```python
from build123d import *

# Parameters (mm, degrees)
F1_ANGLE      = 30
F2_R          = 3.81
F3_DEPTH      = 151.131
F3_DEPTH_BACK = 151.131
F4_W          = 5.08
F4_H          = 20.3206839475
F5_DEPTH      = 2.54


with BuildPart() as f1:
    # F0 (on Top) → F1 (revolve)
    with BuildSketch(Plane.XY):
        with BuildLine():
            Line((-151.13, 0), (-146.05, 0))
            ThreePointArc((-146.05, 0), (0, 146.05), (146.05, 0))
            Line((146.05, 0), (151.13, 0))
            ThreePointArc((151.13, 0), (0, 151.13), (-151.13, 0))
        make_face()
    revolve(axis=Axis((-73.025, 0, 0), (1, 0, 0)), revolution_arc=F1_ANGLE)

    # F2 (on Right) → F3 (cut, two sides)
    with BuildSketch(Plane.YZ) as f3_sk:
        Circle(F2_R)
    extrude(amount=-F3_DEPTH, mode=Mode.SUBTRACT)
    extrude(f3_sk.sketch, amount=F3_DEPTH_BACK, mode=Mode.SUBTRACT)

    # F4 (on Top) → F5 (join)
    with BuildSketch(Plane.XY):
        with Locations((0, 148.5682533469)):
            Rectangle(F4_W, F4_H)
    extrude(amount=F5_DEPTH)


solid = f1.part
```
Work out the finished part from the listing and answer in its coordinate system (mm). Coordinates: 2 decimals unless noted, no trailing zeros. Loops run counter-clockwise (first coordinate to the right, second up) from the corner with the lowest first, then second, coordinate; pieces in that order, holes last. Notation, with made-up numbers: (41.25, 70) - (81.25, 70) arc R33 ccw to (81.25, 107) - close; hole circle Ø2 at (15, -37.75). An arc over 180 degrees is marked (long way). Use a Markdown table: item, result.
Item 1: The mould has two halves that part along Z. Classify faces 1 (the flat face through (-34.279, 124.092, 71.645)), 2 (the flat face through (-1, 139, 0)): +Z half, -Z half, draft (parallel to the pull), parting line (faces both ways), or undercut.
Evaluation:
| item | result |
|---|---|
| face 1 | +Z half |
| face 2 | -Z half |
Item 2: Find section B-B, the plane y = 78. Determine the outline of the cut face in (x, z), and give its area (3 significant figures).
Evaluation:
| item | result |
|---|---|
| outline | (-129.45, 0) - (-123.48, 0) arc R123.48 cw to (-114.97, 45.03) - (-121.36, 45.03) arc R129.45 ccw to start; (114.97, 45.03) arc R123.48 cw to (123.48, 0) - (129.45, 0) arc R129.45 ccw to (121.36, 45.03) - close |
| area | 550 mm2 |
Item 3: Given pin 1 Ø6 at (y, z) = (36.5, 19.5) entering from -X; pin 2 Ø5 at (y, z) = (118.5, 38) entering from +X; pin 3 Ø4 at (x, y) = (1, 141.5) entering from +Z, each flat-ended and moving along its own axis, determine where each tip first touches the part or whether it passes through.
Evaluation:
| item | result |
|---|---|
| pin 1 | stops at x = -146.17 |
| pin 2 | stops at x = 89.27 |
| pin 3 | stops at z = 58.13 |
Item 4: Find section C-C, the plane z = 21. Determine the outline of the cut face in (x, y).
Evaluation:
| item | result |
|---|---|
| outline | (-145.18, 36.37) - (-139.88, 36.37) arc R144.53 cw to (139.88, 36.37) - (145.18, 36.37) arc R149.66 ccw to start |
Item 5: Consider probe 1 along X at (y, z) = (66.5, 12); probe 2 along Y at (x, z) = (-124.5, 31); probe 3 along Y at (x, z) = (3, 3). Determine where each line is inside the solid, lowest interval first. Write a range as from..to.
Evaluation:
| item | result |
|---|---|
| probe 1 | x = -135.18..-129.48, 129.48..135.18 |
| probe 2 | y = 69.78..79.87 |
| probe 3 | y = 145.99..151.07 |
Item 6: Find section A-A, the plane y = 21. Determine the outline of the cut face in (x, z).
Evaluation:
| item | result |
|---|---|
| outline | (-149.66, 0) - (-144.53, 0) arc R144.53 cw to (-144.02, 12.12) - (-149.17, 12.12) arc R149.66 ccw to start; (144.02, 12.12) arc R144.53 cw to (144.53, 0) - (149.66, 0) arc R149.66 ccw to (149.17, 12.12) - close |
Item 7: Find section D-D, the plane x = 31.5. Determine the outline of the cut face in (y, z).
Evaluation:
| item | result |
|---|---|
| outline | (123.51, 71.31) arc R142.61 cw to (142.61, 0) - (147.81, 0) arc R147.81 ccw to (128.01, 73.91) - close |
